Build history of the part. All positions in model axes, mm. A direction names the side the tool comes from. Give positions to 0.01 mm unless a question says otherwise; leave off trailing zeros. Order: outer loops, then holes, each group sorted by start corner. A loop starts at its lowest first (then second) coordinate and runs counter-clockwise, first axis right, second up. Notation, with made-up numbers: (2, 43) - (7, 43) arc R30 ccw to (7, 80) - close; hole circle Ø11 at (-1.75, 29.25). An arc over 180 degrees is marked (long way). Use a Markdown table: item, result. Add a question column.
(1) Slice it at A-A (x = 35). Write the cut outline in (y, z).
(2) Slice it at D-D (z = -5). Write the cut outline in (x, y), then the cut area to 3 significant figures.
(3) Slice it at B-B (z = 7). Write the cut outline in (x, y).
(4) Which spindle directions (+Z, -Z, +X, -X, +Y, -Y) get a long thin tool onto all of the face, cutting with end or side? Do faces 1 (the face through (28, -39, 15.24)), 2 (the face through (37.02, 21, 9)), 3 (the face through (28, 19, 0)). Say none if no direction does.
(5) Slice it at C-C (y = 21). Write the cut outline in (x, z), then the cut area to 3 significant figures.
(6) Wall check: line 1 (Z direction, x = 24.5, y = -39); line 2 (X direction, y = 24.5, z = 12); line 3 (Y direction, x = -0.5, z = 16). Give the ranges that are in metal, low to high.
(7) Mould opens along Y. For faces 4 (the face through (19.286, -18.237, 3.397)), 5 (the face through (-6.336, -28.716, 3.397)), 6 (the face through (28, -15, 19.05)) say: +Y half, -Y half, draft (parallel to the pull), parting line (faces both ways), or undercut.
(8) Flat gauge pins, fed straight in: pin 1 (6.5 mm diameter, centred on y = 21, z = 8, fed in from +X); pin 2 (8 mm diameter, centred on y = -13, z = -8.5, fed in from -X); pin 3 (4 mm diameter, centred on y = -19, z = 7.5, fed in from +X); pin 4 (10 mm diameter, centred on x = -6, y = -32.5, fed in from +Z). Where does each tip first touch, or does it go through?
from build123d import *

# Parameters (mm, degrees)
F1_DEPTH = 19.05
F3_DEPTH = 12.7
F4_DEPTH = 12.7
F5_W     = 3.81
F5_H     = 27.94
F5_W_2   = 20.32
F6_DEPTH = 6.35
F8_DEPTH = 40.386
F9_R     = 6.858


with BuildPart() as f1:
    # F0 (on Top) → F1 (new body)
    with BuildSketch(Plane.XY):
        with BuildLine():
            ThreePointArc((19.2405, 18.2848026719), (24.6498624793, 9.844548174), (26.543, 0))
            ThreePointArc((26.543, 0), (11.6482264852, -23.8505695687), (-16.3195, -20.9333410795))
            Line((-16.3195, -20.9333410795), (3.3713763961, -36.2842234889))
            Line((3.3713763961, -36.2842234889), (52.8896236039, -36.2842234889))
            Line((52.8896236039, -36.2842234889), (72.5805, -20.9333410795))
            ThreePointArc((72.5805, -20.9333410795), (36.597613718, -17.8292481312), (37.0205, 18.2848026719))
            Line((37.0205, 18.2848026719), (19.2405, 18.2848026719))
        make_face()
    extrude(amount=F1_DEPTH)

    # F2 (on face) → F3 (join)
    with BuildSketch(Plane(origin=(0, 0, 0), x_dir=(1, 0, 0), z_dir=(0, 0, -1))):
        with BuildLine():
            ThreePointArc((-16.3195, 20.9333410795), (11.6482264852, 23.8505695687), (26.543, 0))
            Line((26.543, 0), (29.718, 0))
            ThreePointArc((29.718, 0), (44.6127735148, 23.8505695687), (72.5805, 20.9333410795))
            Line((72.5805, 20.9333410795), (52.8896236039, 36.2842234889))
            Line((52.8896236039, 36.2842234889), (3.3713763961, 36.2842234889))
            Line((3.3713763961, 36.2842234889), (-16.3195, 20.9333410795))
        make_face()
    extrude(amount=F3_DEPTH)

    # F4 (add): a face of the model
    f4_faces = [f1.faces().sort_by_distance(p)[0] for p in [
        (28.1305, 18.2848026719, 9.525),
    ]]
    extrude(f4_faces, amount=F4_DEPTH)

    # F5 (on face) → F6 (join)
    with BuildSketch(Plane.XZ.offset(36.2842234889)):
        with Locations((40.1955, 1.27)):
            Rectangle(F5_W, F5_H)
        with Locations((28.1305, 1.27)):
            Rectangle(F5_W_2, F5_H)
        with Locations((16.0655, 1.27)):
            Rectangle(F5_W, F5_H)
    extrude(amount=F6_DEPTH)

    # F7 (on face) → F8 (cut)
    with BuildSketch(Plane(origin=(0, 0, -12.7), x_dir=(1, 0, 0), z_dir=(0, 0, -1))):
        Polygon((42.1005, 42.6342234889), (38.2905, 36.2842234889), (42.1005, 36.2842234889), (42.1005, 42.0675911009), align=None)
        Polygon((17.9705, 36.2842234889), (14.1605, 42.6342234889), (14.1605, 36.2842234889), align=None)
    extrude(amount=-F8_DEPTH, mode=Mode.SUBTRACT)

    # F9
    f9_edges = [f1.edges().sort_by_distance(p)[0] for p in [
        (37.0205, 30.984803, 9.525),
        (19.2405, 30.984803, 9.525),
    ]]
    fillet(f9_edges, radius=F9_R)


solid = f1.part
Solution:
| question | item | result |
|---|---|---|
| 1 | outline | (-42.63, -12.7) - (-15.89, -12.7) - (-15.89, 19.05) - (-36.28, 19.05) - (-36.28, 15.24) - (-42.63, 15.24) - close; (15.89, 0) - (28.99, 0) - (28.99, 19.05) - (15.89, 19.05) - close |
| 2 | outline | (-16.32, -20.93) - (3.37, -36.28) - (17.97, -36.28) - (14.16, -42.63) - (42.1, -42.63) - (38.29, -36.28) - (52.89, -36.28) - (72.58, -20.93) arc R26.54 cw to (29.72, 0) - (26.54, 0) arc R26.54 cw to start |
| 2 | area | 1,160 mm2 |
| 3 | outline | (-16.32, -20.93) - (3.37, -36.28) - (17.97, -36.28) - (14.16, -42.63) - (42.1, -42.63) - (38.29, -36.28) - (52.89, -36.28) - (72.58, -20.93) arc R26.54 cw to (37.02, 18.28) - (37.02, 24.13) arc R6.86 ccw to (30.16, 30.98) - (26.1, 30.98) arc R6.86 ccw to (19.24, 24.13) - (19.24, 18.28) arc R26.54 cw to start |
| 4 | face 1 | +Z, +X, -X, -Y |
| 4 | face 2 | +Z, -Z, +X, +Y |
| 4 | face 3 | -Z, +X, -X, +Y |
| 5 | outline | (19.24, 0) - (37.02, 0) - (37.02, 19.05) - (19.24, 19.05) - close |
| 5 | area | 339 mm2 |
| 6 | line 1 | -12.7 to 15.24 |
| 6 | line 2 | 19.25 to 37.01 |
| 6 | line 3 | -33.27 to -26.54 |
| 7 | face 4 | undercut |
| 7 | face 5 | -Y half |
| 7 | face 6 | draft |
| 8 | pin 1 | x = 37.02 |
| 8 | pin 2 | x = 20.38 |
| 8 | pin 3 | x = 72.58 |
| 8 | pin 4 | z = 19.05 |
